Here's how the part is built. I have some questions about the finished solid (model axes, mm). Face numbers are marked on the shaded views. A direction names the side the tool comes from. Give positions to 0.01 mm unless a question says otherwise; leave off trailing zeros. Loops run counter-clockwise (first coordinate to the right, second up) from the corner with the lowest first, then second, coordinate; pieces in that order, holes last. Notation, with made-up numbers: (-0.75, 35.5) - (19.25, 35.5) arc R7 cw to (19.25, 41.5) - close; hole circle Ø7 at (30.25, 46.5). An arc over 180 degrees is marked (long way). Use one line per item in the form item = value.
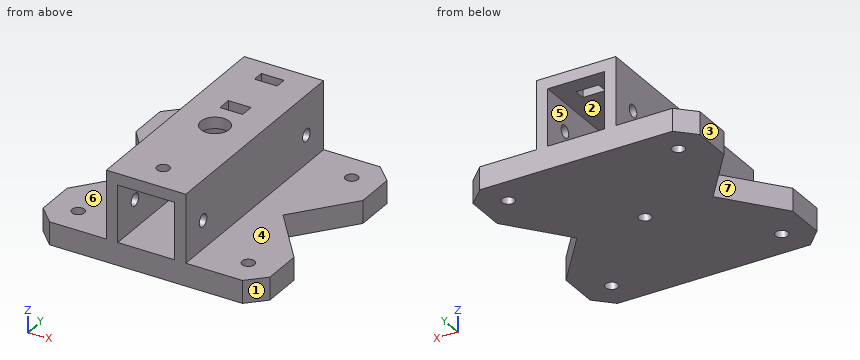
from build123d import *

# Parameters (mm, degrees)
ESQUISSE1_W             = 80
ESQUISSE1_H             = 80
BOSS_EXTRU_1_DEPTH      = 8
ESQUISSE2_W             = 28
ESQUISSE2_H             = 28
ESQUISSE2_W_2           = 20
ESQUISSE2_H_2           = 20
BOSS_EXTRU_2_DEPTH      = 80
D_GAGEMENT_M41_D        = 4.4
D_GAGEMENT_M42_D        = 4.4
D_GAGEMENT_M101_D       = 10
D_GAGEMENT_M101_DEPTH   = 28
D_GAGEMENT_M43_D        = 4.4
D_GAGEMENT_M43_DEPTH    = 5
ESQUISSE13_W            = 8
ESQUISSE13_H            = 4
ESQUISSE13_H_2          = 4.898494306
ENL_V_MAT_EXTRU_1_DEPTH = 4
ENL_V_MAT_EXTRU_2_DEPTH = 9
CHANFREIN2_SIZE         = 6


with BuildPart() as part:
    # Esquisse1 → Boss.-Extru.1 (new body)
    with BuildSketch(Plane.XY):
        Rectangle(ESQUISSE1_W, ESQUISSE1_H)
    extrude(amount=BOSS_EXTRU_1_DEPTH)

    # Esquisse2 → Boss.-Extru.2 (add, through all)
    with BuildSketch(Plane(origin=(0, 40, 0), x_dir=(1, 0, 0), z_dir=(0, 1, 0))):
        with Locations((0, -18)):
            Rectangle(ESQUISSE2_W, ESQUISSE2_H)
        with Locations((0, -18)):
            Rectangle(ESQUISSE2_W_2, ESQUISSE2_H_2, mode=Mode.SUBTRACT)
    extrude(amount=-BOSS_EXTRU_2_DEPTH)

    # Dégagement M41 (through all)
    with Locations(Plane(origin=(0, 0, 0), x_dir=(-1, 0, 0), z_dir=(0, 0, -1))):
        with Locations((-30, 30), (30, 30), (30, -30), (-30, -30), (0, 0)):
            Hole(D_GAGEMENT_M41_D / 2)

    # Dégagement M42 (through all)
    with Locations(Plane(origin=(14, 0, 0), x_dir=(0, 0, -1), z_dir=(1, 0, 0))):
        with Locations((-18, 30), (-18, -30)):
            Hole(D_GAGEMENT_M42_D / 2)

    # Dégagement M101
    with Locations(Plane.XY.offset(32)):
        with Locations((0, 0)):
            Hole(D_GAGEMENT_M101_D / 2, depth=D_GAGEMENT_M101_DEPTH)

    # Dégagement M43
    with Locations(Plane.XY.offset(32)):
        with Locations((0, -30)):
            Hole(D_GAGEMENT_M43_D / 2, depth=D_GAGEMENT_M43_DEPTH)

    # Esquisse13 → Enlèv. mat.-Extru.1 (cut)
    with BuildSketch(Plane.XY.offset(32)):
        with Locations((-0.307514137, 32)):
            Rectangle(ESQUISSE13_W, ESQUISSE13_H)
        with Locations((-0.307514137, 12.405785937)):
            Rectangle(ESQUISSE13_W, ESQUISSE13_H_2)
    extrude(amount=-ENL_V_MAT_EXTRU_1_DEPTH, mode=Mode.SUBTRACT)

    # Esquisse14 → Enlèv. mat.-Extru.2 (cut, through all)
    with BuildSketch(Plane.XY.offset(8)):
        Polygon((-40, 20), (-24, 0), (-40, -20), align=None)
        Polygon((40, 20), (24, 0), (40, -20), align=None)
    extrude(amount=-ENL_V_MAT_EXTRU_2_DEPTH, mode=Mode.SUBTRACT)

    # Chanfrein2
    chanfrein2_edges = [part.edges().sort_by_distance(p)[0] for p in [
        (40, -40, 4),
        (-40, -40, 4),
        (-40, 40, 4),
        (40, 40, 4),
    ]]
    chamfer(chanfrein2_edges, length=CHANFREIN2_SIZE)


solid = part.part
(1) If I drill on probe 1 along Y at (x, z) = (0, 29.1); probe 2 along Y at (x, z) = (12.25, 18); probe 3 along Y at (x, z) = (0, 5), over which ranges is the centre line in solid material (lowest first)?
Geometry says:
probe_1 = -40 to -32.2, -27.8 to -5, 5 to 9.96, 14.86 to 30, 34 to 40
probe_2 = -40 to -32.2, -27.8 to 27.8, 32.2 to 40
probe_3 = -40 to -5, 5 to 40
(2) For the marked faces 4, 5, 6 and 7, which set-ups out of +Z, -Z, +X, -X, +Y, -Y let a thin tool reach every point of the face, with its end or its side?
Geometry says:
face_4 = +Z, +X, +Y, -Y
face_5 = +Y, -Y
face_6 = +Z, -X, +Y, -Y
face_7 = +Z, -Z, -X
(3) If we section it at A-A (x = 0): Give the number of separate pieces and of enclosed holes in the cut face, plus the area to 3 significant figures.
Geometry says:
separate_pieces = 7
enclosed_holes = 0
area = 809 mm²
(4) For P1, Ø1.2, axis at y = 32, z = 29.5, coming from the -X side; P2, Ø4, axis at x = -12, y = 28.5, coming from the -Z side; P3, Ø5, axis at x = 30, y = 30, coming from the +Z side; P4, Ø12, axis at y = 5.5, z = 10.5, coming from the +X side, each with a flat end and sliding along its axis, tell me the tip position at first contact or that it passes through.
Geometry says:
P1 = -14
P2 = 0
P3 = 8
P4 = 32.76
(5) If we section it at B-B (z = 11): List the corners of the cut face in (x, y) for me, plus the area to 3 significant figures.
Geometry says:
outline = (-14, -40) - (-10, -40) - (-10, 40) - (-14, 40) - close; (10, -40) - (14, -40) - (14, 40) - (10, 40) - close
area = 640 mm²
(6) If we section it at D-D (z = 18): List the corners of the cut face in (x, y) for me, plus the area to 3 significant figures.
Geometry says:
outline = (-14, -40) - (-10, -40) - (-10, -32.2) - (-14, -32.2) - close; (-14, -27.8) - (-10, -27.8) - (-10, 27.8) - (-14, 27.8) - close; (-14, 32.2) - (-10, 32.2) - (-10, 40) - (-14, 40) - close; (10, -40) - (14, -40) - (14, -32.2) - (10, -32.2) - close; (10, -27.8) - (14, -27.8) - (14, 27.8) - (10, 27.8) - close; (10, 32.2) - (14, 32.2) - (14, 40) - (10, 40) - close
area = 570 mm²
(7) Thinking about a two-plate mould opening in X: for the marked faces 1, 2 and 3, which applies, pulls with the +X half, pulls with the -X half, needs draft (parallel to the pull), parting line crosses it, or undercut?
Geometry says:
face_1 = pulls with the +X half
face_2 = undercut
face_3 = pulls with the -X half
(8) If we section it at C-C (y = -24.5): List the corners of the cut face in (x, z) for me, plus the area to 3 significant figures.
Geometry says:
outline = (-40, 0) - (40, 0) - (40, 8) - (14, 8) - (14, 32) - (-14, 32) - (-14, 8) - (-40, 8) - close; hole (-10, 8) - (10, 8) - (10, 28) - (-10, 28) - close
area = 912 mm²
